Source: three-view drawing plus pictorial views. Frame: mm from the lowest corner of the part. Give positions to 0.01 mm unless a question says otherwise; leave off trailing zeros. Loops run counter-clockwise (first coordinate to the right, second up) from the corner with the lowest first, then second, coordinate; pieces in that order, holes last.
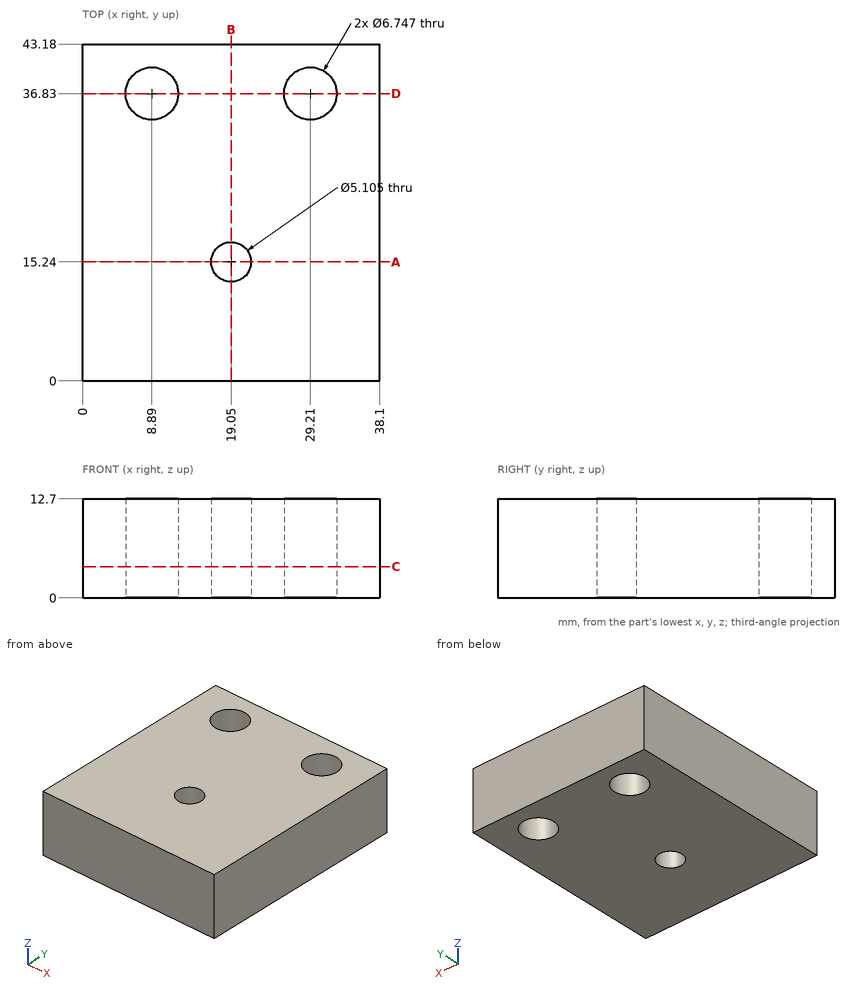
Q1. Section query D-D, the plane y = 36.83. Return loops of the section in (x, z).
Q2. Material intervals for probe 1 along X at (y, z) = (38, 6.25) (1 decimal); probe 2 along Y at (x, z) = (19.05, 4); probe 3 along Y at (x, z) = (8.89, 9.5), sorted ascending.
Q3. Section query B-B, the plane x = 19.05. Return loops of the section in (y, z).
Q4. Section query A-A, the plane y = 15.24. Return loops of the section in (x, z), and give its area (3 significant figures).
Q5. Section query C-C, the plane z = 4. State how many separate pieces and enclosed holes the cut face has, and give its area (3 significant figures).
Resolved:
1. outline: (0, 0) - (5.52, 0) - (5.52, 12.7) - (0, 12.7) - close; (12.26, 0) - (25.84, 0) - (25.84, 12.7) - (12.26, 12.7) - close; (32.58, 0) - (38.1, 0) - (38.1, 12.7) - (32.58, 12.7) - close
2. probe 1: x = 0 to 5.7, 12.1 to 26, 32.4 to 38.1
2. probe 2: y = 0 to 12.69, 17.79 to 43.18
2. probe 3: y = 0 to 33.46, 40.2 to 43.18
3. outline: (0, 0) - (12.69, 0) - (12.69, 12.7) - (0, 12.7) - close; (17.79, 0) - (43.18, 0) - (43.18, 12.7) - (17.79, 12.7) - close
4. outline: (0, 0) - (16.5, 0) - (16.5, 12.7) - (0, 12.7) - close; (21.6, 0) - (38.1, 0) - (38.1, 12.7) - (21.6, 12.7) - close
4. area: 419 mm2
5. separate pieces: 1
5. enclosed holes: 3
5. area: 1,550 mm2
